Design review of the part built by this model. Coordinates are the model's own, in mm. Give positions to 0.01 mm unless a question says otherwise; leave off trailing zeros. Write each loop counter-clockwise with the first axis right and the second up, starting at its lowest first coordinate (ties: lowest second). Pieces come first, ordered by that corner, then holes. Notation, with made-up numbers: (-4, -27) -> (35, -27) arc R7 cw to (35, -19) -> close; hole circle Ø11 at (-19.5, -18.5). An arc over 180 degrees is marked (long way). Answer as a JSON object with one key per item and string values.
```python
from build123d import *

# Parameters (mm, degrees)
SKETCH1_R           = 3.333333333
BOSS_EXTRUDE1_DEPTH = 635
FILLET4_R           = 0.508


with BuildPart() as part:
    # Sketch1 → Boss-Extrude1 (new body)
    with BuildSketch(Plane(origin=(0, 0, 0), x_dir=(1, 0, 0), z_dir=(0, 1, 0))):
        Polygon((4.285, 17.618333333), (6.666666667, 20), (0, 20), (0, 13.333333333), (2.381666667, 15.715), (2.381666667, 4.285), (0, 6.666666667), (0, 0), (6.666666667, 0), (4.285, 2.381666667), (15.715, 2.381666667), (13.333333333, 0), (20, 0), (20, 6.666666667), (17.618333333, 4.285), (17.618333333, 15.715), (20, 13.333333333), (20, 20), (13.333333333, 20), (15.715, 17.618333333), align=None)
        with Locations((10, 10)):
            Circle(SKETCH1_R, mode=Mode.SUBTRACT)
    extrude(amount=BOSS_EXTRUDE1_DEPTH)

    # Fillet4
    fillet4_edges = [part.edges().sort_by_distance(p)[0] for p in [
        (20, 317.5, 0),
        (0, 317.5, 0),
        (0, 317.5, -20),
        (20, 317.5, -20),
    ]]
    fillet(fillet4_edges, radius=FILLET4_R)


solid = part.part
```
(1) For line 1 along Z through (x, y) = (10, 236); line 2 along Z through (x, y) = (15.25, 428.5); line 3 along Z through (x, y) = (6, 194), list the stretches that pass through material, from the lowest coordinate up.
Here are the results:
{"line 1": "z = -17.62 to -13.33, -6.67 to -2.38", "line 2": "z = -20 to -18.08, -17.62 to -2.38, -1.92 to 0", "line 3": "z = -20 to -19.33, -17.62 to -2.38, -0.67 to 0"}
(2) We need section C-C, the plane y = 101. State the section outline as (x, z) points (3 decimals).
Here are the results:
{"outline": "(0, -19.492) arc R0.508 ccw to (0.508, -20) -> (6.667, -20) -> (4.285, -17.618) -> (15.715, -17.618) -> (13.333, -20) -> (19.492, -20) arc R0.508 ccw to (20, -19.492) -> (20, -13.333) -> (17.618, -15.715) -> (17.618, -4.285) -> (20, -6.667) -> (20, -0.508) arc R0.508 ccw to (19.492, 0) -> (13.333, 0) -> (15.715, -2.382) -> (4.285, -2.382) -> (6.667, 0) -> (0.508, 0) arc R0.508 ccw to (0, -0.508) -> (0, -6.667) -> (2.382, -4.285) -> (2.382, -15.715) -> (0, -13.333) -> close; hole circle Ø6.667 at (10, -10)"}
(3) We need section B-B, the plane x = 10. State the section outline as (y, z) points.
Here are the results:
{"outline": "(0, -17.62) -> (635, -17.62) -> (635, -13.33) -> (0, -13.33) -> close; (0, -6.67) -> (635, -6.67) -> (635, -2.38) -> (0, -2.38) -> close"}
(4) Clearance check with flat-ended pins moving along their axes: pin 1 (5.5 mm diameter, centred on x = 10, z = -10, fed in from +Y); pin 2 (3.5 mm diameter, centred on x = 8.5, y = 252, fed in from +Z). State where each tip first meets the part, or that it passes through.
Here are the results:
{"pin 1": "passes through", "pin 2": "stops at z = -2.38"}
(5) We need section A-A, the plane z = -10. State the section outline as (x, y) points, then the cut area to 3 significant figures.
Here are the results:
{"outline": "(2.38, 0) -> (6.67, 0) -> (6.67, 635) -> (2.38, 635) -> close; (13.33, 0) -> (17.62, 0) -> (17.62, 635) -> (13.33, 635) -> close", "area": "5,440 mm²"}
(6) The part is to be moulded in two halves that separate along Z. For faces 1 (the flat face through (5, 0, -10)), 2 (the flat face through (2.382, 313, -10)), say which applies: +Z half, -Z half, draft (parallel to the pull), parting line (faces both ways), or undercut.
Here are the results:
{"face 1": "draft", "face 2": "undercut"}
